Source: CAD feature listing. Evaluate the final solid. Frame: model axes, mm. Face numbers are marked on the shaded views. Round coordinates to 2 decimals unless told otherwise and drop trailing zeros. Loops run counter-clockwise (first coordinate to the right, second up) from the corner with the lowest first, then second, coordinate; pieces in that order, holes last.
Item 1: Section query C-C on y = 9. Give the number of separate pieces and of enclosed holes in the cut face, then the cut area to 3 significant figures.
Item 2: Pull-direction query (Z, two-part tool) for the marked faces 1 and 2; classes: released by +Z, released by -Z, zero draft, split by the parting line, or undercut.
Item 3: Section query B-B on z = -39. Return loops of the section in (x, y), then the cut area to 3 significant figures.
Item 4: Ray query, L1, parallel to Z at x = -1.5, y = 12; L2, parallel to Z at x = -44.5, y = 10.25; L3, parallel to X at y = 10.5, z = -24.5. Return the intervals inside material, ascending.
Item 5: Section query A-A on x = 7. Return loops of the section in (y, z), then the cut area to 3 significant figures.
```python
from build123d import *

# Parameters (mm, degrees)
EXTRUDE_1_DEPTH     = 14
SKETCH_3_R          = 1.7
CUT_EXTRUDE_1_DEPTH = 118.45637488
SKETCH_4_R          = 3.4
CUT_EXTRUDE_2_DEPTH = 118.45637488
SKETCH_5_R          = 16.999999997
CUT_EXTRUDE_3_DEPTH = 118.45637488
SKETCH_6_R          = 4
CUT_EXTRUDE_4_DEPTH = 118.45637488


with BuildPart() as part:
    # 草图1 → 凸台-拉伸1 (new body)
    with BuildSketch(Plane(origin=(0, 0, 0), x_dir=(1, 0, 0), z_dir=(0, 1, 0))):
        with BuildLine():
            Line((-57, -100), (57, -100))
            ThreePointArc((57, -100), (59.121320344, -99.121320344), (60, -97))
            Line((60, -97), (60, 57))
            ThreePointArc((60, 57), (59.121320344, 59.121320344), (57, 60))
            Line((57, 60), (-57, 60))
            ThreePointArc((-57, 60), (-59.121320344, 59.121320344), (-60, 57))
            Line((-60, 57), (-60, -97))
            ThreePointArc((-60, -97), (-59.121320344, -99.121320344), (-57, -100))
        make_face()
    extrude(amount=EXTRUDE_1_DEPTH)

    # 草图3 → 切除-拉伸1 (cut, through all)
    with BuildSketch(Plane.XZ):
        with Locations(Location((14.849242405, -24.150757595, 0), (0, 0, 270))):
            Circle(SKETCH_3_R)
        with Locations(Location((14.849242405, -53.849242405, 0), (0, 0, 270))):
            Circle(SKETCH_3_R)
        with Locations(Location((-14.849242405, -53.849242405, 0), (0, 0, 270))):
            Circle(SKETCH_3_R)
        with Locations(Location((-14.849242405, -24.150757595, 0), (0, 0, 270))):
            Circle(SKETCH_3_R)
    extrude(amount=-CUT_EXTRUDE_1_DEPTH, mode=Mode.SUBTRACT)

    # 草图4 → 切除-拉伸2 (cut, through all)
    with BuildSketch(Plane.XZ):
        with Locations(Location((0, 85, 0), (0, 0, 270))):
            Circle(SKETCH_4_R)
        with Locations(Location((45, 40, 0), (0, 0, 270))):
            Circle(SKETCH_4_R)
        with Locations(Location((-45, 40, 0), (0, 0, 270))):
            Circle(SKETCH_4_R)
    extrude(amount=-CUT_EXTRUDE_2_DEPTH, mode=Mode.SUBTRACT)

    # 草图5 → 切除-拉伸3 (cut, through all)
    with BuildSketch(Plane(origin=(0, 14, 0), x_dir=(1, 0, 0), z_dir=(0, 1, 0))):
        with Locations(Location((4e-09, 38.999999996, 0), (0, 0, 270))):
            Circle(SKETCH_5_R)
    extrude(amount=-CUT_EXTRUDE_3_DEPTH, mode=Mode.SUBTRACT)

    # 草图6 → 切除-拉伸4 (cut, through all)
    with BuildSketch(Plane.XZ):
        with Locations(Location((40, 80, 0), (0, 0, 270))):
            Circle(SKETCH_6_R)
        with Locations(Location((-40, 80, 0), (0, 0, 90))):
            Circle(SKETCH_6_R)
        with Locations(Location((40, -40, 0), (0, 0, 90))):
            Circle(SKETCH_6_R)
        with Locations(Location((-40, -40, 0), (0, 0, 270))):
            Circle(SKETCH_6_R)
    extrude(amount=-CUT_EXTRUDE_4_DEPTH, mode=Mode.SUBTRACT)


solid = part.part
```
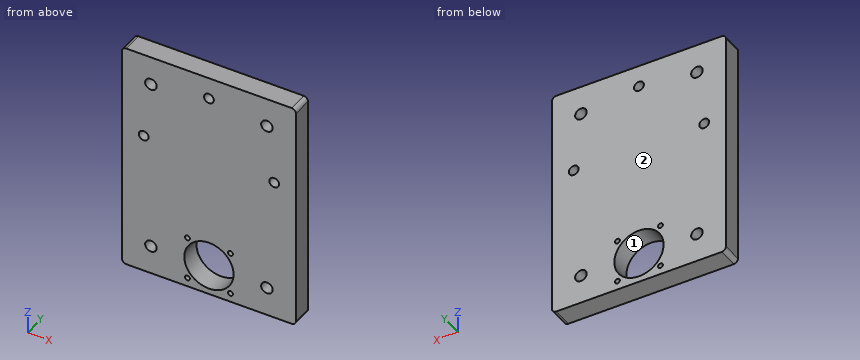
Data:
1. separate pieces: 1
1. enclosed holes: 12
1. area: 17,900 mm2
2. face 1: undercut
2. face 2: zero draft
3. outline: (-60, 0) - (-43.87, 0) - (-43.87, 14) - (-60, 14) - close; (-36.13, 0) - (-17, 0) - (-17, 14) - (-36.13, 14) - close; (17, 0) - (36.13, 0) - (36.13, 14) - (17, 14) - close; (43.87, 0) - (60, 0) - (60, 14) - (43.87, 14) - close
3. area: 987 mm2
4. L1: z = -60 to -55.93, -22.07 to 81.95, 88.05 to 100
4. L2: z = -60 to 36.64, 43.36 to 100
4. L3: x = -60 to -16.51, -13.19 to -8.87, 8.87 to 13.19, 16.51 to 60
5. outline: (0, -60) - (14, -60) - (14, -54.49) - (0, -54.49) - close; (0, -23.51) - (14, -23.51) - (14, 100) - (0, 100) - close
5. area: 1,810 mm2
